from build123d import *

# Parameters (mm, degrees)
F0_W      = 113.0752004683
F0_H      = 11.9665954262
F1_DEPTH  = 60
F3_DEPTH  = 12
F5_W      = 12.1646374464
F5_H      = 59.8628073931
F6_DEPTH  = 60
F4_W      = 49.9786976725
F4_H      = 20.8079274744
F7_DEPTH  = 50
F9_DEPTH  = 21
F10_R     = 12.6598002667
F11_DEPTH = 21


with BuildPart() as f1:
    # F0 (on Front) → F1 (new body)
    with BuildSketch(Plane.XZ):
        with Locations((-12.968538329, 5.9832977131)):
            Rectangle(F0_W, F0_H)
    extrude(amount=F1_DEPTH)

    # F2 (on face) → F3 (cut)
    with BuildSketch(Plane.XY.offset(11.9665954262)):
        Polygon((43.5690619051, -60), (-69.5061385632, -20.8079274744), (-69.5061385632, -60), align=None)
    extrude(amount=-F3_DEPTH, mode=Mode.SUBTRACT)

    # F5 (on Top) → F6 (join)
    with BuildSketch(Plane.XY):
        with Locations((49.6189072728, -29.9314036965)):
            Rectangle(F5_W, F5_H)
    extrude(amount=F6_DEPTH)

    # F4 (on face) → F7 (join)
    with BuildSketch(Plane.XY.offset(11.9665954262)):
        with Locations((-44.5167897269, -10.4039637372)):
            Rectangle(F4_W, F4_H)
    extrude(amount=F7_DEPTH)

    # F8 (on face) → F9 (cut)
    with BuildSketch(Plane.XZ.offset(20.8079274744)):
        with BuildLine():
            ThreePointArc((-69.5061385632, 36.9665954262), (-44.5167897269, 61.9559442624), (-19.5274408907, 36.9665954262))
            Line((-19.5274408907, 36.9665954262), (-19.5274408907, 61.9665954262))
            Line((-19.5274408907, 61.9665954262), (-69.5061385632, 61.9665954262))
            Line((-69.5061385632, 61.9665954262), (-69.5061385632, 36.9665954262))
        make_face()
    extrude(amount=-F9_DEPTH, mode=Mode.SUBTRACT)

    # F10 (on face) → F11 (cut)
    with BuildSketch(Plane.XZ.offset(20.8079274744)):
        with Locations((-44.5167897269, 36.9665954262)):
            Circle(F10_R)
    extrude(amount=-F11_DEPTH, mode=Mode.SUBTRACT)


solid = f1.part
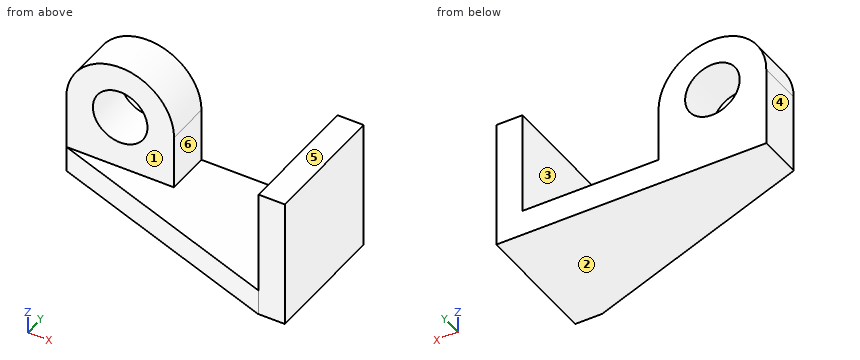
Build history of the part. All positions in model axes, mm. Face numbers are marked on the shaded views. A direction names the side the tool comes from. Give positions to 0.01 mm unless a question says otherwise; leave off trailing zeros. Order: outer loops, then holes, each group sorted by start corner. A loop starts at its lowest first (then second) coordinate and runs counter-clockwise, first axis right, second up. Notation, with made-up numbers: M -6,23.25 L 6,23.25 A22 cw 6,37.25 Z; hole C 34,-22.75 d7. An arc over 180 degrees is marked long. Use one line per item in the form item = value.
Q1. Which spindle directions (+Z, -Z, +X, -X, +Y, -Y) get a long thin tool onto all of the face, cutting with end or side? Do the marked faces 1, 2 and 3. Say none if no direction does.
Conclusion:
face_1 = +Z, -X, -Y
face_2 = -Z, +X, -X, +Y, -Y
face_3 = +Z, +Y, -Y
Q2. Slice it at C-C, the plane z = 52.5. Write the cut outline in (x, y), and give its area (3 significant figures).
Conclusion:
outline = M -64.09,-20.81 L -24.94,-20.81 L -24.94,0 L -64.09,0 Z; M 43.54,-59.86 L 55.7,-59.86 L 55.7,0 L 43.54,0 Z
area = 1,540 mm2
Q3. Wall check: probe 1 along X at (y, z) = (-8, 37); probe 2 along X at (y, z) = (-19, 13); probe 3 along X at (y, z) = (-5, 38). Give the ranges that are in metal, low to high.
Conclusion:
probe_1 = -69.51 to -57.18, -31.86 to -19.53, 43.54 to 55.7
probe_2 = -69.51 to -19.53, 43.54 to 55.7
probe_3 = -69.48 to -57.13, -31.9 to -19.55, 43.54 to 55.7
Q4. Pull direction X, two halves, no side cores. Call the marked faces 4, 5 and 6: released by +X, released by -X, zero draft, split by the parting line, or undercut.
Conclusion:
face_4 = released by -X
face_5 = zero draft
face_6 = undercut
Q5. Slice it at D-D, the plane z = 31. Write the cut outline in (x, y).
Conclusion:
outline = M -69.51,-20.81 L -55.68,-20.81 L -55.68,0 L -69.51,0 Z; M -33.35,-20.81 L -19.53,-20.81 L -19.53,0 L -33.35,0 Z; M 43.54,-59.86 L 55.7,-59.86 L 55.7,0 L 43.54,0 Z
Q6. Pin check, flat tips, straight feed: P1, Ø20.5, axis at x = -44.52, z = 36.97, coming from the +Y side; P2, Ø18, axis at x = -23, y = -16, coming from the +Z side; P3, Ø4, axis at x = -31.5, z = 38, coming from the -Y side; P4, Ø13.5, axis at x = 52, y = -27.5, coming from the +Z side. Stop position of each tip, or through.
Conclusion:
P1 = through
P2 = 58.6
P3 = -20.81
P4 = 60
Q7. Slice it at A-A, the plane x = -52.5. Write the cut outline in (y, z), and give its area (3 significant figures).
Conclusion:
outline = M -26.7,0 L 0,0 L 0,27.14 L -20.81,27.14 L -20.81,11.97 L -26.7,11.97 Z; M -20.81,46.79 L 0,46.79 L 0,60.65 L -20.81,60.65 Z
area = 924 mm2
Q8. Slice it at B-B, the plane y = -11. Write the cut outline in (x, z).
Conclusion:
outline = M -69.51,0 L 55.7,0 L 55.7,60 L 43.54,60 L 43.54,11.97 L -19.53,11.97 L -19.53,36.97 A24.99 ccw -69.51,36.97 Z; hole C -44.52,36.97 d25.32
